Geometry: final body of the model. Coordinates: model frame, mm. Face numbers are marked on the shaded views. Give positions to 0.01 mm unless a question says otherwise; leave off trailing zeros. Write each loop counter-clockwise with the first axis right and the second up, starting at its lowest first coordinate (ties: lowest second). Pieces come first, ordered by that corner, then holes. Notation, with made-up numbers: M 34.25,13 L 57.25,13 A9 ccw 57.25,23 Z; hole C 70.5,53.5 d2. An arc over 180 degrees is marked long. Use a Markdown table: item, result. Add a question column.
(1) Material intervals for L1, parallel to X at y = 1.75, z = 0; L2, parallel to X at y = 3.25, z = 11.5; L3, parallel to X at y = 2.25, z = -12.5, sorted ascending.
(2) Pin query (flat end, axial travel): pin 1 Ø2 at (x, y) = (11, 1.5) entering from +Z; pin 2 Ø1.9 at (x, z) = (-22, -12.7) entering from +Y; pin 3 Ø1 at (y, z) = (4, -6) entering from +X. Return the tip coordinate at first contact, or that it passes through.
(3) Draft query along Z for the marked faces 1 and 2. Return one class per face: released by +Z, released by -Z, zero draft, split by the parting line, or undercut.
(4) Cut plane D-D (z = -21). Output: boundary loops of the cut face in (x, y) (3 decimals).
(5) Cut plane B-B (x = 0). State how many separate pieces and enclosed holes the cut face has, plus the area to 3 significant figures.
(6) Cut plane C-C (z = 12.7). Output: boundary loops of the cut face in (x, y) (3 decimals), plus the area to 3 significant figures.
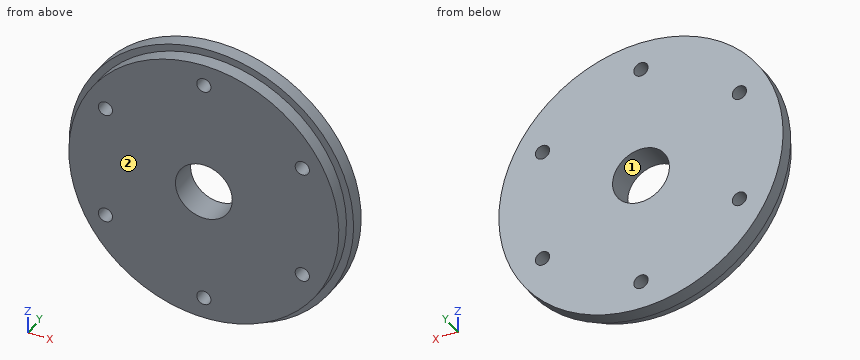
```python
from build123d import *

# Parameters (mm, degrees)
SKETCH1_R           = 30.1625
BOSS_EXTRUDE1_DEPTH = 3.175
SKETCH2_R           = 31.75
BOSS_EXTRUDE2_DEPTH = 3.175
SKETCH3_R           = 1.5875
SKETCH3_R_2         = 6.35
CUT_EXTRUDE1_DEPTH  = 46.348070521


with BuildPart() as part:
    # Sketch1 → Boss-Extrude1 (new body)
    with BuildSketch(Plane(origin=(0, 0, 0), x_dir=(1, 0, 0), z_dir=(0, 1, 0))):
        with Locations(Location((0, 0, 0), (0, 0, 270))):
            Circle(SKETCH1_R)
    extrude(amount=BOSS_EXTRUDE1_DEPTH)

    # Sketch2 → Boss-Extrude2 (add)
    with BuildSketch(Plane(origin=(0, 3.175, 0), x_dir=(1, 0, 0), z_dir=(0, 1, 0))):
        with Locations(Location((0, 0, 0), (0, 0, 270))):
            Circle(SKETCH2_R)
    extrude(amount=BOSS_EXTRUDE2_DEPTH)

    # Sketch3 → Cut-Extrude1 (cut, through all)
    with BuildSketch(Plane(origin=(0, 6.35, 0), x_dir=(1, 0, 0), z_dir=(0, 1, 0))):
        with Locations(Location((0, 25.4, 0), (0, 0, 270))):
            Circle(SKETCH3_R)
        with Locations(Location((21.997045256, 12.7, 0), (0, 0, 270))):
            Circle(SKETCH3_R)
        with Locations(Location((21.997045256, -12.7, 0), (0, 0, 270))):
            Circle(SKETCH3_R)
        with Locations(Location((0, -25.4, 0), (0, 0, 270))):
            Circle(SKETCH3_R)
        with Locations(Location((-21.997045256, -12.7, 0), (0, 0, 270))):
            Circle(SKETCH3_R)
        with Locations(Location((-21.997045256, 12.7, 0), (0, 0, 270))):
            Circle(SKETCH3_R)
        with Locations(Location((0, 0, 0), (0, 0, 270))):
            Circle(SKETCH3_R_2)
    extrude(amount=-CUT_EXTRUDE1_DEPTH, mode=Mode.SUBTRACT)


solid = part.part
```
Answer list:
| question | item | result |
|---|---|---|
| 1 | L1 | -30.16 to -6.35, 6.35 to 30.16 |
| 1 | L2 | -29.59 to -23.04, -20.96 to 20.96, 23.04 to 29.59 |
| 1 | L3 | -27.45 to -23.57, -20.42 to 20.42, 23.57 to 27.45 |
| 2 | pin 1 | z = 28.46 |
| 2 | pin 2 | through |
| 2 | pin 3 | x = 31.27 |
| 3 | face 1 | undercut |
| 3 | face 2 | zero draft |
| 4 | outline | M -23.813,3.175 L -21.651,3.175 L -21.651,0 L 21.651,0 L 21.651,3.175 L 23.813,3.175 L 23.813,6.35 L -23.813,6.35 Z |
| 5 | separate pieces | 4 |
| 5 | enclosed holes | 0 |
| 5 | area | 272 mm² |
| 6 | outline | M -29.099,3.175 L -27.358,3.175 L -27.358,0 L -23.585,0 L -23.585,6.35 L -29.099,6.35 Z; M -20.41,0 L 20.41,0 L 20.41,6.35 L -20.41,6.35 Z; M 23.585,0 L 27.358,0 L 27.358,3.175 L 29.099,3.175 L 29.099,6.35 L 23.585,6.35 Z |
| 6 | area | 318 mm² |
